from build123d import *

# Parameters (mm, degrees)
BOSS_EXTRUDE1_DEPTH     = 1.3
SKETCH2_R               = 2.5
SKETCH2_R_2             = 1.79
BOSS_EXTRUDE2_DEPTH     = 5
CUT_EXTRUDE1_DEPTH      = 11.942298947
CUT_EXTRUDE1_DEPTH_BACK = 11.942298947
SKETCH4_R               = 1.79


with BuildPart() as part:
    # Sketch1 → Boss-Extrude1 (new body)
    with BuildSketch(Plane.XY):
        with BuildLine():
            ThreePointArc((-2.327269665, 3.784131765), (-9.2625, 0), (-2.327269665, -3.784131765))
            ThreePointArc((-2.327269665, -3.784131765), (0, -3.1), (2.327269665, -3.784131765))
            ThreePointArc((2.327269665, -3.784131765), (9.2625, 0), (2.327269665, 3.784131765))
            ThreePointArc((2.327269665, 3.784131765), (0, 3.1), (-2.327269665, 3.784131765))
        make_face()
    boss_extrude1 = extrude(amount=BOSS_EXTRUDE1_DEPTH)

    # Sketch2 → Boss-Extrude2 (add)
    # profile 1 of 2: a face of its own
    with BuildSketch(Plane.XY.offset(1.3)):
        with Locations(Location((-4.7625, 0, 0), (0, 0, 180))):
            Circle(SKETCH2_R)
        with Locations((-4.7625, 0)):
            Circle(SKETCH2_R_2, mode=Mode.SUBTRACT)
    # profile 2 of 2: a face of its own
    with BuildSketch(Plane.XY.offset(1.3)):
        with Locations(Location((4.7625, 0, 0), (0, 0, 180))):
            Circle(SKETCH2_R)
        with Locations((4.7625, 0)):
            Circle(SKETCH2_R_2, mode=Mode.SUBTRACT)
    extrude(amount=BOSS_EXTRUDE2_DEPTH)

    # Mirror5: Boss-Extrude1 across plane
    add(boss_extrude1.mirror(Plane(origin=(0, 0, 3.7), x_dir=(1, 0, 0), z_dir=(0, 0, -1))))

    # Sketch4 → Cut-Extrude1 (cut, two sides: drawn at the far end of the back side and taken through both)
    with BuildSketch(Plane(origin=(0, 0, 3.7), x_dir=(-1, 0, 0), z_dir=(0, 0, -1)).offset(-CUT_EXTRUDE1_DEPTH_BACK)):
        with Locations((-4.7625, 0)):
            Circle(SKETCH4_R)
        with Locations((4.7625, 0)):
            Circle(SKETCH4_R)
    extrude(amount=CUT_EXTRUDE1_DEPTH + CUT_EXTRUDE1_DEPTH_BACK, mode=Mode.SUBTRACT)


solid = part.part
CAD build for the part. Positions are in the model's coordinates, mm. A direction names the side the tool comes from. Give positions to 0.01 mm unless a question says otherwise; leave off trailing zeros. Order: outer loops, then holes, each group sorted by start corner. A loop starts at its lowest first (then second) coordinate and runs counter-clockwise, first axis right, second up. Notation, with made-up numbers: (16, 45) - (51, 45) arc R27 ccw to (51, 75) - close; hole circle Ø11 at (-10, 89.5). An arc over 180 degrees is marked (long way). Answer in a Markdown table with one row per item.
1. Saw through at B-B, the plane y = -2.75. Give the cut face in (x, z), plus the area to 3 significant figures.
Data:
| item | result |
|---|---|
| outline | (-8.32, 0) - (8.32, 0) - (8.32, 1.3) - (-8.32, 1.3) - close; (-8.32, 6.1) - (8.32, 6.1) - (8.32, 7.4) - (-8.32, 7.4) - close |
| area | 43.3 mm² |
2. Saw through at C-C, the plane x = 4.75. Give the cut face in (y, z), plus the area to 3 significant figures.
Data:
| item | result |
|---|---|
| outline | (-4.5, 0) - (-1.79, 0) - (-1.79, 7.4) - (-4.5, 7.4) - (-4.5, 6.1) - (-2.5, 6.1) - (-2.5, 1.3) - (-4.5, 1.3) - close; (1.79, 0) - (4.5, 0) - (4.5, 1.3) - (2.5, 1.3) - (2.5, 6.1) - (4.5, 6.1) - (4.5, 7.4) - (1.79, 7.4) - close |
| area | 20.9 mm² |
3. Probe probe 1 along X at (y, z) = (0, 0.75); probe 2 along Y at (x, z) = (-4.75, 3.5); probe 3 along Z at (x, y) = (-5.25, 3.75). List the from-to ranges inside material, lowest first. Write a range as [from, to].
Data:
| item | result |
|---|---|
| probe 1 | x = [-9.26, -6.55], [-2.97, 2.97], [6.55, 9.26] |
| probe 2 | y = [-2.5, -1.79], [1.79, 2.5] |
| probe 3 | z = [0, 1.3], [6.1, 7.4] |
4. Pull direction X, two halves, no side cores. Call faces 3 (the cylindrical face through (9.26, -0.13, 6.76)), 4 (the flat face through (0, 0, 7.4)), 5 (the cylindrical face through (0, -3.1, 6.8)): pulls with the +X half, pulls with the -X half, needs draft (parallel to the pull), parting line crosses it, or undercut.
Data:
| item | result |
|---|---|
| face 3 | undercut |
| face 4 | needs draft |
| face 5 | undercut |
5. Saw through at A-A, the plane z = 2.5. Give the cut face in (x, y), plus the area to 3 significant figures.
Data:
| item | result |
|---|---|
| outline | circle Ø5 at (-4.76, 0); circle Ø5 at (4.76, 0); hole circle Ø3.58 at (-4.76, 0); hole circle Ø3.58 at (4.76, 0) |
| area | 19.1 mm² |
6. Tool access for faces 1 (the cylindrical face through (0, 3.1, 0.6)), 2 (the cylindrical face through (-7.07, 0.96, 3.67)): list every direction of +Z, -Z, +X, -X, +Y, -Y with a clear straight run to the whole face (end or side of a thin tool).
Data:
| item | result |
|---|---|
| face 1 | +Z, -Z, +Y |
| face 2 | none |
7. Flat gauge pins, fed straight in: pin 1 (1 mm diameter, centred on x = 2.5, y = -0.5, fed in from -Z); pin 2 (1 mm diameter, centred on x = 3.5, z = 2, fed in from -Y). Where does each tip first touch, or does it go through?
Data:
| item | result |
|---|---|
| pin 1 | stops at z = 0 |
| pin 2 | stops at y = -2.38 |
